For this review, take the finished solid that the model builds, in its own axes (mm). A direction names the side the tool comes from. Give positions to 0.01 mm unless a question says otherwise; leave off trailing zeros. Order: outer loops, then holes, each group sorted by start corner. A loop starts at its lowest first (then second) coordinate and runs counter-clockwise, first axis right, second up.
from build123d import *

# Parameters (mm, degrees)
F3_D            = 10
F3_COPIES_COUNT = 4


# Not quite as in the source:
# - a pattern or mirror of a feature is missing from the dataset's text; its kind, count and spacing are read off the source's solid


with BuildPart() as f1:
    # F0 (on Top) → F1 (revolve)
    with BuildSketch(Plane.XY):
        Polygon((42.5, 60.944458911), (9, 60.944458911), (9, -24.055541089), (14, -24.055541089), (19.277993122, 12.944458911), (19.277993122, 42.944458911), (42.5, 42.944458911), align=None)
    revolve(axis=Axis((0, 17.8779862242, 0), (0, -1, 0)))

    # F3 (through all)
    with Locations(Plane.XZ.offset(-42.944458911)):
        with Locations((32.5, 0)):
            f3 = Hole(F3_D / 2)

    # F3_copies: F3 ×4 about axis
    f3_copies_axis = Axis((0, 0, 0), (0, 1, 0))
    for i in range(1, F3_COPIES_COUNT):
        add(f3.rotate(f3_copies_axis, i * 360 / F3_COPIES_COUNT), mode=Mode.SUBTRACT)


solid = f1.part
1) To check wall thickness, follow line 1 (Z direction, x = -3, y = 52); line 2 (Y direction, x = -34, z = 11.5); line 3 (Z direction, x = 0, y = -2). State the ranges of each line that lie inside material, in increasing order.
Answer sheet:
line 1: z = -42.39 to -36.5, -28.5 to -8.49, 8.49 to 28.5, 36.5 to 42.39
line 2: y = 42.94 to 60.94
line 3: z = -17.15 to -9, 9 to 17.15
2) We need section D-D on z = -32.5. Give the boundary of the cut face in (x, y), then the cut area to 3 significant figures.
Answer sheet:
outline: (-27.39, 42.94) - (-5, 42.94) - (-5, 60.94) - (-27.39, 60.94) - close; (5, 42.94) - (27.39, 42.94) - (27.39, 60.94) - (5, 60.94) - close
area: 806 mm2
3) We need section C-C on y = 52. Give the boundary of the cut face in (x, z).
Answer sheet:
outline: circle Ø85 at (0, 0); hole circle Ø10 at (-32.5, 0); hole circle Ø18 at (0, 0); hole circle Ø10 at (0, -32.5); hole circle Ø10 at (0, 32.5); hole circle Ø10 at (32.5, 0)
4) Draft analysis for pull direction Z (two halves, no side actions). For faces 1 (the face through (18.39, 28.15, 5.79)), 2 (the face through (-0.22, 52.07, 37.495)), 3 (the face through (-10, 60.944, 1)), state which applies: +Z half, -Z half, draft (parallel to the pull), parting line (faces both ways), or undercut.
Answer sheet:
face 1: parting line
face 2: undercut
face 3: draft
5) Tool access review of faces 4 (the face through (19.5, 42.944, 0.6)), 5 (the face through (-1.172, 17.849, 8.923)): name each direction out of +Z, -Z, +X, -X, +Y, -Y from which nothing blocks a thin tool from reaching the whole face with its end or side.
Answer sheet:
face 4: -Y
face 5: +Y, -Y
6) Clearance check with flat-ended pins moving along their axes: pin 1 (8 mm diameter, centred on y = -5.5, z = -13, fed in from +X); pin 2 (10 mm diameter, centred on x = 6, y = -3.5, fed in from -Z); pin 3 (1.5 mm diameter, centred on x = -26.5, z = 3.5, fed in from -Y). State where each tip first meets the part, or that it passes through.
Answer sheet:
pin 1: stops at x = 14.09
pin 2: stops at z = -17.26
pin 3: stops at y = 42.94
7) We need section A-A on z = 0. Give the boundary of the cut face in (x, y), then the cut area to 3 significant figures.
Answer sheet:
outline: (-42.5, 42.94) - (-37.5, 42.94) - (-37.5, 60.94) - (-42.5, 60.94) - close; (-27.5, 42.94) - (-19.28, 42.94) - (-19.28, 12.94) - (-14, -24.06) - (-9, -24.06) - (-9, 60.94) - (-27.5, 60.94) - close; (9, -24.06) - (14, -24.06) - (19.28, 12.94) - (19.28, 42.94) - (27.5, 42.94) - (27.5, 60.94) - (9, 60.94) - close; (37.5, 42.94) - (42.5, 42.94) - (42.5, 60.94) - (37.5, 60.94) - close
area: 2,030 mm2
8) We need section B-B on x = -32.5. Give the boundary of the cut face in (y, z), then the cut area to 3 significant figures.
Answer sheet:
outline: (42.94, -27.39) - (60.94, -27.39) - (60.94, -5) - (42.94, -5) - close; (42.94, 5) - (60.94, 5) - (60.94, 27.39) - (42.94, 27.39) - close
area: 806 mm2
